Read the model definition and answer for the solid it produces. Units are mm, in the model's axes. A direction names the side the tool comes from. Give positions to 0.01 mm unless a question says otherwise; leave off trailing zeros. Use a Markdown table: item, result.
from build123d import *

# Parameters (mm, degrees)
BOSS_EXTRUDE1_DEPTH = 6.35
SKETCH2_W           = 43.7
SKETCH2_H           = 43.7
CUT_EXTRUDE1_DEPTH  = 2.54
CUT_EXTRUDE3_DEPTH  = 2.54
SKETCH4_W           = 2.8
SKETCH4_H           = 7.7
SKETCH4_W_2         = 7.7
SKETCH4_H_2         = 33.528
CUT_EXTRUDE4_DEPTH  = 2.54
CUT_EXTRUDE6_DEPTH  = 165.648464375
CUT_EXTRUDE7_DEPTH  = 1.5
SKETCH9_W           = 50
SKETCH9_H           = 10.5
CUT_EXTRUDE8_DEPTH  = 2.54


with BuildPart() as part:
    # Sketch1 → Boss-Extrude1 (new body)
    with BuildSketch(Plane(origin=(0, 0, 0), x_dir=(1, 0, 0), z_dir=(0, 1, 0))):
        with BuildLine():
            Line((52.544610399, 96), (92.384610399, 96))
            ThreePointArc((92.384610399, 96), (95.976712847, 94.512102448), (97.464610399, 90.92))
            Line((97.464610399, 90.92), (97.464610399, 57.942930422))
            add(Edge.make_bspline(
                [(127.445958891, -2.757399797), (126.217398064, 6.772879157), (124.527871566, 26.937506289), (103.198818931, 39.120916323), (97.37297865, 51.416446236), (97.464610399, 57.942930422)],
                knots=[0, 0, 0, 0, 0.4542014, 0.725733713, 1, 1, 1, 1], degree=3))
            add(Edge.make_bspline(
                [(127.445958891, -2.757399797), (127.822967418, -13.097877655), (122.880457127, -26.665652965), (112.775276891, -43.705151038), (101.21628269, -54.346897272), (78.643551493, -67.273421727), (58.317264726, -71.917502632), (43.855300998, -72.741727337)],
                knots=[0, 0, 0, 0, 0.251847695, 0.354064973, 0.49200618, 0.63769577, 1, 1, 1, 1], degree=3))
            Line((43.855300998, -72.741727337), (39.503738361, -72.784901588))
            ThreePointArc((39.503738361, -72.784901588), (36.074693376, -74.391591034), (34.256026209, -77.71307417))
            ThreePointArc((34.256026209, -77.71307417), (34.316151416, -80.336736497), (35.431566201, -82.712250947))
            ThreePointArc((35.431566201, -82.712250947), (37.591781392, -87.927471757), (35.431566201, -93.142692568))
            add(Edge.make_bspline(
                [(35.431566201, -93.142692568), (33.316240589, -95.95188132), (29.837032497, -99.83422186), (25.835087368, -103.598548459), (24, -104.01567246)],
                knots=[0, 0, 0, 0, 0.654699401, 1, 1, 1, 1], degree=3))
            add(Edge.make_bspline(
                [(12.568433799, -93.142692568), (14.683759411, -95.95188132), (18.162967503, -99.83422186), (22.164912632, -103.598548459), (24, -104.01567246)],
                knots=[0, 0, 0, 0, 0.654699401, 1, 1, 1, 1], degree=3))
            ThreePointArc((12.568433799, -93.142692568), (10.408218608, -87.927471757), (12.568433799, -82.712250947))
            ThreePointArc((12.568433799, -82.712250947), (13.683848584, -80.336736497), (13.743973791, -77.71307417))
            ThreePointArc((13.743973791, -77.71307417), (11.925306624, -74.391591034), (8.496261639, -72.784901588))
            Line((8.496261639, -72.784901588), (4.144699002, -72.741727337))
            add(Edge.make_bspline(
                [(-79.445958891, -2.757399797), (-79.822967418, -13.097877655), (-74.880457127, -26.665652965), (-64.775276891, -43.705151038), (-53.21628269, -54.346897272), (-30.643551493, -67.273421727), (-10.317264726, -71.917502632), (4.144699002, -72.741727337)],
                knots=[0, 0, 0, 0, 0.251847695, 0.354064973, 0.49200618, 0.63769577, 1, 1, 1, 1], degree=3))
            add(Edge.make_bspline(
                [(-79.445958891, -2.757399797), (-78.217398064, 6.772879157), (-76.527871566, 26.937506289), (-55.198818931, 39.120916323), (-49.37297865, 51.416446236), (-49.464610399, 57.942930422)],
                knots=[0, 0, 0, 0, 0.4542014, 0.725733713, 1, 1, 1, 1], degree=3))
            Line((-49.464610399, 57.942930422), (-49.464610399, 90.92))
            ThreePointArc((-49.464610399, 90.92), (-47.976712847, 94.512102448), (-44.384610399, 96))
            Line((-44.384610399, 96), (-4.544610399, 96))
            ThreePointArc((-4.544610399, 96), (-0.95250795, 94.512102448), (0.535389601, 90.92))
            Line((0.535389601, 90.92), (0.535389601, 56.693089242))
            ThreePointArc((0.535389601, 56.693089242), (3.823086605, 49.0674139), (11.540006197, 46))
            Line((11.540006197, 46), (36.459993803, 46))
            ThreePointArc((36.459993803, 46), (44.176913395, 49.0674139), (47.464610399, 56.693089242))
            Line((47.464610399, 56.693089242), (47.464610399, 90.92))
            ThreePointArc((47.464610399, 90.92), (48.95250795, 94.512102448), (52.544610399, 96))
        make_face()
    extrude(amount=BOSS_EXTRUDE1_DEPTH)

    # Sketch2 → Cut-Extrude1 (cut)
    with BuildSketch(Plane(origin=(0, 6.35, 0), x_dir=(1, 0, 0), z_dir=(0, 1, 0))):
        with Locations((-24.114610399, 70.15)):
            Rectangle(SKETCH2_W, SKETCH2_H)
        with Locations((24.69959658, -8.994026969)):
            Rectangle(SKETCH2_W, SKETCH2_H)
        Polygon((91.756041109, 22.663971871), (61.687394919, -8.87), (93.287751095, -39.001945738), (123.356397284, -7.467973867), align=None)
        Polygon((-44.043312702, -39.001945738), (-74.111958891, -7.467973867), (-42.511602716, 22.663971871), (-12.442956526, -8.87), align=None)
    extrude(amount=-CUT_EXTRUDE1_DEPTH, mode=Mode.SUBTRACT)

    # Sketch5 → Cut-Extrude3 (cut)
    with BuildSketch(Plane(origin=(0, 6.35, 0), x_dir=(1, 0, 0), z_dir=(0, 1, 0))):
        Polygon((104.769890137, 10.254852474), (122.226588264, 28.562262267), (128.147086585, 23.613346709), (110.342548256, 4.94114553), align=None)
        Polygon((11.522520215, 48.786329059), (-29.825516941, 9.359659151), (-24.511809997, 3.787001032), (16.836227159, 43.213670941), (19.758341498, 46), align=None)
    extrude(amount=-CUT_EXTRUDE3_DEPTH, mode=Mode.SUBTRACT)

    # Sketch4 → Cut-Extrude4 (cut)
    with BuildSketch(Plane(origin=(0, 6.35, 0), x_dir=(1, 0, 0), z_dir=(0, 1, 0))):
        with Locations((-0.864610399, 70.15)):
            Rectangle(SKETCH4_W, SKETCH4_H)
        with Locations((24.700041109, 29.236)):
            Rectangle(SKETCH4_W_2, SKETCH4_H_2)
    extrude(amount=-CUT_EXTRUDE4_DEPTH, mode=Mode.SUBTRACT)

    # Sketch6 → Cut-Extrude6 (cut, through all)
    with BuildSketch(Plane(origin=(0, 6.35, 0), x_dir=(1, 0, 0), z_dir=(0, 1, 0))):
        with BuildLine():
            Line((86.506282583, 36.458848797), (69.305686566, 14.862795995))
            ThreePointArc((69.305686566, 14.862795995), (57.802795593, 14.587410011), (59.565699046, 25.95774464))
            Line((59.565699046, 25.95774464), (83.207643636, 40.216372063))
            Line((83.207643636, 40.216372063), (86.506282583, 36.458848797))
        make_face()
        with BuildLine():
            Line((-10.890245417, -21.894543883), (-9.654995767, -22.825371259))
            Line((-9.654995767, -22.825371259), (-22.640520119, -48.35628634))
            ThreePointArc((-22.640520119, -48.35628634), (-33.316925376, -50.071712063), (-34.61076845, -39.336057229))
            Line((-34.61076845, -39.336057229), (-13.648173317, -19.816296144))
            Line((-13.648173317, -19.816296144), (-12.475776388, -20.699760598))
            Line((-12.475776388, -20.699760598), (-10.890245417, -21.894543883))
        make_face()
    extrude(amount=-CUT_EXTRUDE6_DEPTH, mode=Mode.SUBTRACT)

    # Sketch8 → Cut-Extrude7 (cut)
    with BuildSketch(Plane(origin=(0, 6.35, 0), x_dir=(1, 0, 0), z_dir=(0, 1, 0))):
        with BuildLine():
            ThreePointArc((-10.298257622, -20.773023834), (-4.271120984, -10.022070609), (-2.051088275, 2.101494298))
            ThreePointArc((-2.051088275, 2.101494298), (0.822630209, 18.715850278), (8.785888639, 33.577936193))
            Line((8.785888639, 33.577936193), (15.212793605, 41.665675358))
            Line((15.212793605, 41.665675358), (6.835409986, 33.67757335))
            ThreePointArc((6.835409986, 33.67757335), (-1.127848444, 18.815487435), (-4.001566928, 2.201131456))
            ThreePointArc((-4.001566928, 2.201131456), (-6.191058386, -10.025989743), (-12.251111868, -20.869057457))
            Line((-12.251111868, -20.869057457), (-11.052607664, -21.772195154))
            Line((-11.052607664, -21.772195154), (-10.298257622, -20.773023834))
        make_face()
        Polygon((85.351758952, 37.77398194), (102.619850578, 52.933222628), (101.470052745, 53.919838498), (84.362167268, 38.90123892), align=None)
    extrude(amount=-CUT_EXTRUDE7_DEPTH, mode=Mode.SUBTRACT)

    # Sketch9 → Cut-Extrude8 (cut)
    with BuildSketch(Plane(origin=(0, 6.35, 0), x_dir=(1, 0, 0), z_dir=(0, 1, 0))):
        with Locations((72.464610399, 71.7)):
            Rectangle(SKETCH9_W, SKETCH9_H)
    extrude(amount=-CUT_EXTRUDE8_DEPTH, mode=Mode.SUBTRACT)


solid = part.part
Item 1: Straight lines are drawn through the part: line 1 along X through (y, z) = (5, -63.5); line 2 along X through (y, z) = (5, -6.5); line 3 along Z through (x, y) = (37, 5). For each, find the intervals that lie inside material, in ascending order. Write a range as [from, to].
Return value:
| item | result |
|---|---|
| line 1 | [-49.46, -45.96], [-2.26, 0.54], [47.46, 97.46] |
| line 2 | [-78.23, -59.46], [-21.67, -3.78], [-1.82, 2.85], [46.55, 76.34], [111.83, 126.23] |
| line 3 | [-46.01, -12.86], [30.84, 73.68], [85.03, 90.82] |
Item 2: Each of these flat-tipped pins is pushed along its axis until it touches: P1, Ø1, axis at y = 5, z = -31, coming from the +X side; P2, Ø3, axis at y = 1, z = -68.5, coming from the +X side; P3, Ø12, axis at x = 79.5, z = -63, coming from the -Y side; P4, Ø1.3, axis at x = 66, y = 5, coming from the +Z side. Where does it stop, or does it pass through?
Return value:
| item | result |
|---|---|
| P1 | x = 116.02 |
| P2 | x = 97.46 |
| P3 | y = 0 |
| P4 | z = 69.61 |
Item 3: For a pull along X with two mould halves and no side action, classify faces 1 (the face through (116.94, 5.1, 1.35)), 2 (the face through (34.308, 3.131, 80.301)), 3 (the face through (78.026, 3.219, -25.812)), 4 (the face through (72, 3, -96)) as +X half, -X half, draft (parallel to the pull), parting line (faces both ways), or undercut.
Return value:
| item | result |
|---|---|
| face 1 | undercut |
| face 2 | +X half |
| face 3 | undercut |
| face 4 | draft |
Item 4: A tool of negligible diameter and unlimited length cuts with its end or side. For faces 5 (the face through (116.97, 5.1, -11.89)), 6 (the face through (72, 3.81, -72)), 7 (the face through (-24.276, 3.219, 29.713)), from which of +Z, -Z, +X, -X, +Y, -Y can it reach the whole face along a straight path? Write none if from no direction.
Return value:
| item | result |
|---|---|
| face 5 | +Y |
| face 6 | +X, +Y |
| face 7 | +Y, -Y |
Item 5: A cutting plane is placed at A-A (y = 1). Count the separate pieces of the cut face and the enclosed holes in it, then the cut area to 3 significant figures.
Return value:
| item | result |
|---|---|
| separate pieces | 1 |
| enclosed holes | 2 |
| area | 26,100 mm^2 |
